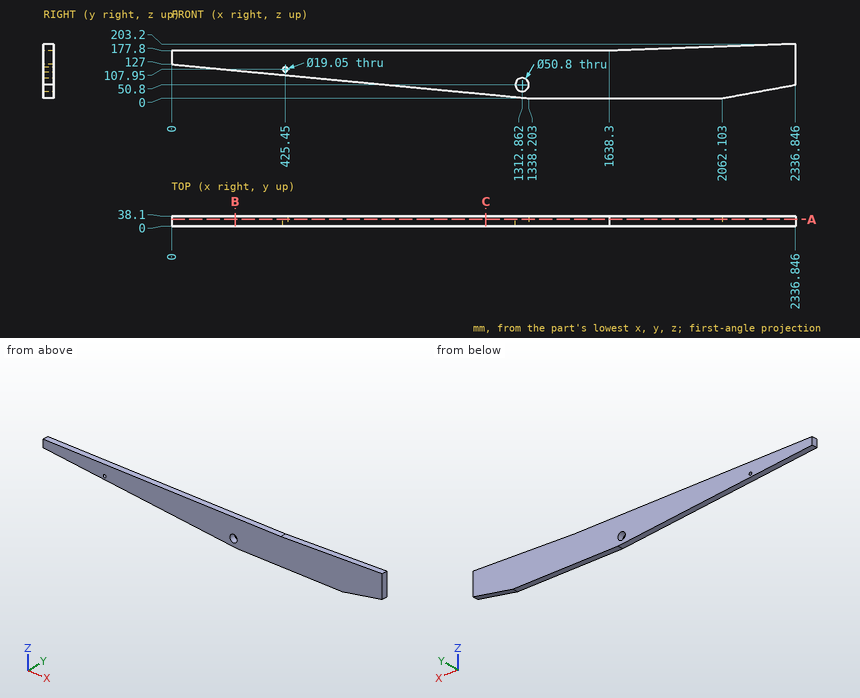
Answer from the drawing. Dimensions are ordinates in mm from the lowest x, y and z of the part. Give positions to 0.01 mm unless a question says otherwise; leave off trailing zeros. Write each loop counter-clockwise with the first axis right and the second up, starting at its lowest first coordinate (ties: lowest second). Pieces come first, ordered by that corner, then holes. Notation, with made-up numbers: (85, 36) - (141, 36) arc R35 ccw to (141, 74) - close; hole circle Ø3 at (41, -29). An arc over 180 degrees is marked (long way). One line per item, written item: value. Start each with the question number.
1. Find section B-B (x = 238). Write down the section's boundary in (y, z), then the cut area to 3 significant figures.
2. Find section C-C (x = 1177). Write down the section's boundary in (y, z), then the cut area to 3 significant figures.
3. Given pin 1 (8 mm diameter, centred on x = 692.5, y = 9, fed in from +Z); pin 2 (8 mm diameter, centred on x = 955, y = 18.5, fed in from -Z), each flat-ended and moving along its own axis, determine where each tip first touches the part or whether it passes through.
4. Consider probe 1 along Z at (x, y) = (1614, 17.5); probe 2 along Z at (x, y) = (425.45, 16.5) (1 decimal); probe 3 along Z at (x, y) = (875, 23.5). Determine where each line is inside the solid, lowest interval first.
5. Find section A-A (y = 26.5). State how many separate pieces and enclosed holes the cut face has, then the cut area to 3 significant figures.
Geometry results:
1. outline: (0, 104.41) - (38.1, 104.41) - (38.1, 177.8) - (0, 177.8) - close
1. area: 2,800 mm2
2. outline: (0, 15.3) - (38.1, 15.3) - (38.1, 177.8) - (0, 177.8) - close
2. area: 6,190 mm2
3. pin 1: z = 177.8
3. pin 2: z = 35.99
4. probe 1: 0 to 177.8
4. probe 2: 86.6 to 98.4, 117.5 to 177.8
4. probe 3: 43.96 to 177.8
5. separate pieces: 1
5. enclosed holes: 2
5. area: 330,000 mm2
